Here's the drawing with two shaded views (mm, measured from the low corner). I have some questions. A direction names the side the tool comes from. Give positions to 0.01 mm unless a question says otherwise; leave off trailing zeros. Loops run counter-clockwise (first coordinate to the right, second up) from the corner with the lowest first, then second, coordinate; pieces in that order, holes last. Notation, with made-up numbers: (-32.75, 87) - (11.25, 87) arc R32 ccw to (11.25, 113) - close; hole circle Ø5 at (49, 53.25). An arc over 180 degrees is marked (long way). Answer as a JSON object with one key per item and string values. Group by question number.
Item 1: Thinking about a two-plate mould opening in X: for the marked faces 1, 2, 3 and 4, which applies, pulls with the +X half, pulls with the -X half, needs draft (parallel to the pull), parting line crosses it, or undercut?
Item 2: Suppose I cut it at C-C on y = 33. Write out the boundary of the cut face in (x, z).
Item 3: Suppose I cut it at A-A on x = 4. Count the separate pieces of the cut face and the enclosed holes in it, and give its area (3 significant figures).
Item 4: Suppose I cut it at B-B on z = 0.75. Write out the boundary of the cut face in (x, y), and give its area (3 significant figures).
Item 5: Which directions (+Z, -Z, +X, -X, +Y, -Y) give clear straight access to the entire face, cutting with the end or side of a thin tool? Please do the marked faces 5 and 6.
Item 6: Will these pins go through, and if not, where does the flat tip stop? pin 1 (3 mm diameter, centred on x = 5.5, z = 6.5, fed in from +Y); pin 2 (2.5 mm diameter, centred on x = 5.5, y = 21.5, fed in from +Z); pin 3 (3.5 mm diameter, centred on x = 4, y = 33, fed in from -Z).
Item 7: Please list where these lines run through material, in increasing order: L1, parallel to Y at x = 4, z = 1.5; L2, parallel to Z at x = 2, y = 28; L3, parallel to Y at x = 6.75, z = 1.25.
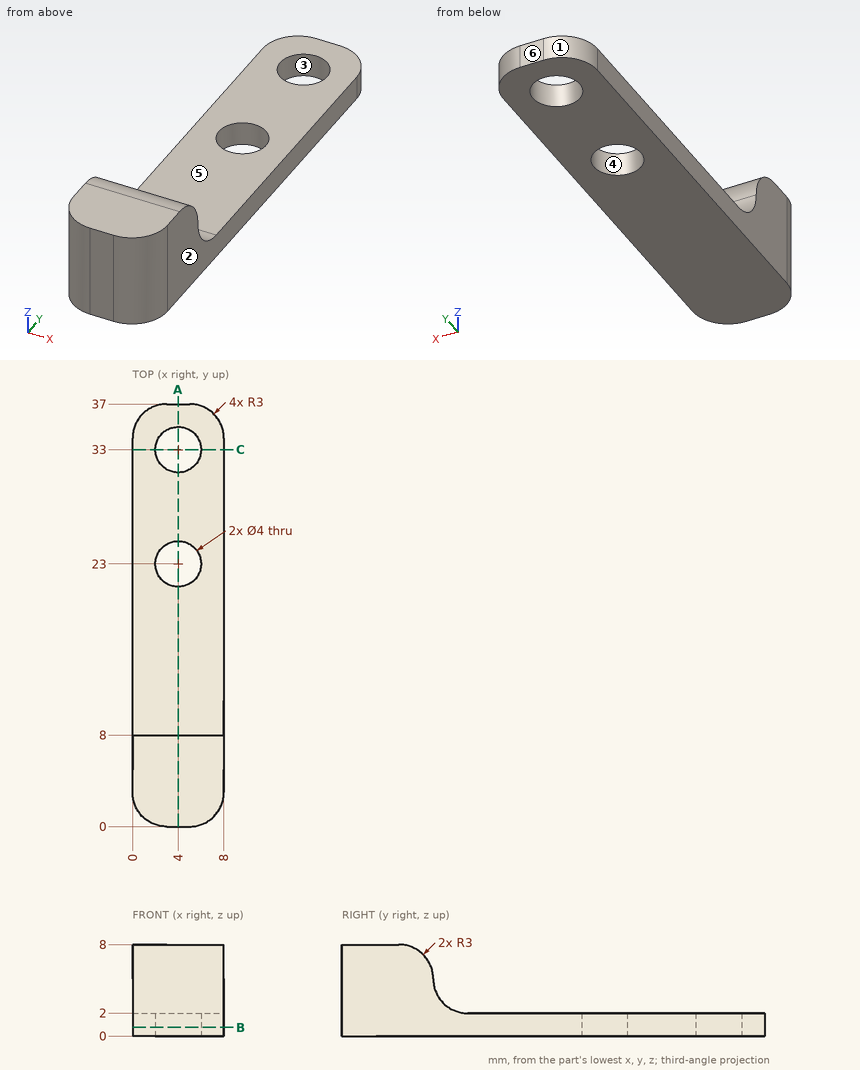
Worked out:
{
 "1": {"face 1": "pulls with the -X half", "face 2": "pulls with the +X half", "face 3": "undercut", "face 4": "undercut"},
 "2": {"outline": "(0, 0) - (2, 0) - (2, 2) - (0, 2) - close; (6, 0) - (8, 0) - (8, 2) - (6, 2) - close"},
 "3": {"separate pieces": "3", "enclosed holes": "0", "area": "106 mm2"},
 "4": {"outline": "(0, 3) arc R3 ccw to (3, 0) - (5, 0) arc R3 ccw to (8, 3) - (8, 34) arc R3 ccw to (5, 37) - (3, 37) arc R3 ccw to (0, 34) - close; hole circle Ø4 at (4, 23); hole circle Ø4 at (4, 33)", "area": "263 mm2"},
 "5": {"face 5": "+Z, +X, -X, +Y", "face 6": "+Z, -Z, +X, -X, +Y"},
 "6": {"pin 1": "stops at y = 8", "pin 2": "stops at z = 2", "pin 3": "passes through"},
 "7": {"L1": "y = 0 to 21, 25 to 31, 35 to 37", "L2": "z = 0 to 2", "L3": "y = 0.56 to 36.44"}
}
